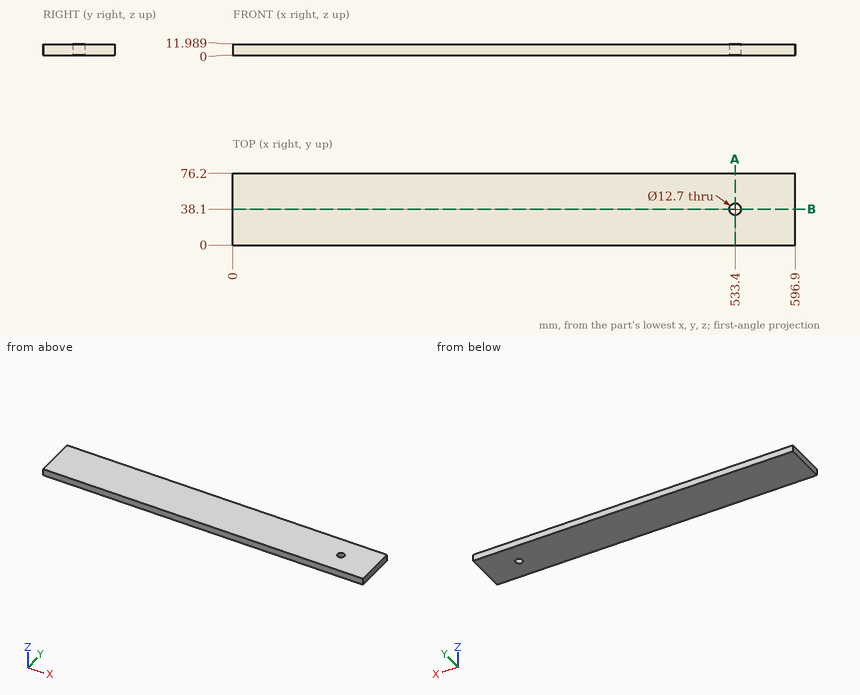
Part print with two shaded views. Sizes in mm from the minimum x, y, z corner. Round coordinates to 2 decimals unless told otherwise and drop trailing zeros. Loops run counter-clockwise (first coordinate to the right, second up) from the corner with the lowest first, then second, coordinate; pieces in that order, holes last. Notation, with made-up numbers: M -3.5,44.25 L 38.5,44.25 A14 cw 38.5,50.25 Z; hole C -33,81 d4. An arc over 180 degrees is marked long. Put each result on its own line as item: value. Start each with the question number.
Item 1: Cut at A-A (x = 533.4). List the corners of the cut face in (y, z).
Item 2: Drill centre lines: line 1 along X through (y, z) = (38.1, 3); line 2 along Y through (x, z) = (533.4, 8.25); line 3 along X through (y, z) = (40, 8.5). Where is each one in solid material? Low to high.
Item 3: Cut at B-B (y = 38.1). List the corners of the cut face in (x, z), then the cut area to 3 significant figures.
Answer block:
1. outline: M 0,0 L 31.75,0 L 31.75,11.99 L 0,11.99 Z; M 44.45,0 L 76.2,0 L 76.2,11.99 L 44.45,11.99 Z
2. line 1: 0 to 527.05, 539.75 to 596.9
2. line 2: 0 to 31.75, 44.45 to 76.2
2. line 3: 0 to 527.34, 539.46 to 596.9
3. outline: M 0,0 L 527.05,0 L 527.05,11.99 L 0,11.99 Z; M 539.75,0 L 596.9,0 L 596.9,11.99 L 539.75,11.99 Z
3. area: 7,000 mm2
